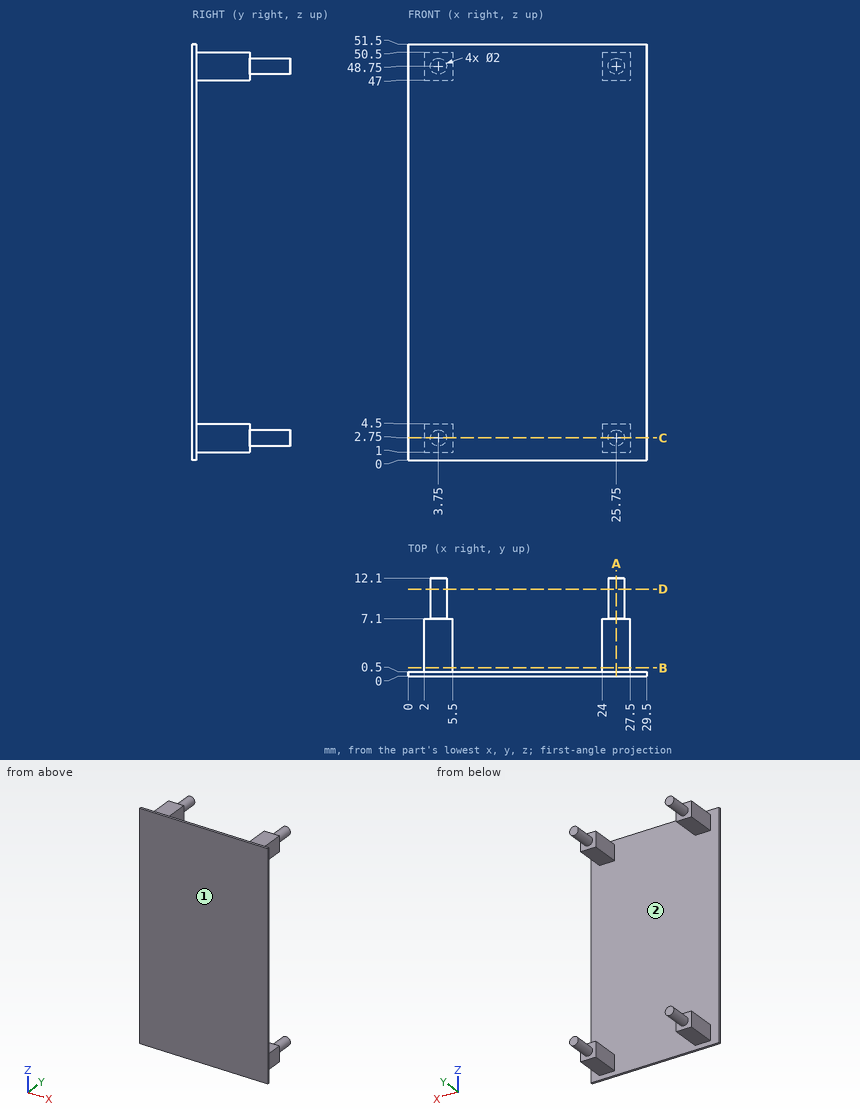
For this review, use the dimensioned drawing (mm, ordinates from the lowest corner) and the shaded views. Coordinates: 2 decimals unless noted, no trailing zeros. Write each loop counter-clockwise with the first axis right and the second up, starting at its lowest first coordinate (ties: lowest second). Pieces come first, ordered by that corner, then holes. Notation, with made-up numbers: (89, 0.25) - (98, 0.25) arc R28 ccw to (98, 25.25) - close; hole circle Ø8 at (-18, 26.5). An arc over 180 degrees is marked (long way). Answer in a Markdown table with one row per item. Add a question column.
Q1. Consider section C-C on z = 2.75. Give the boundary of the cut face in (x, y).
Q2. Clearance check with flat-ended pins moving along their axes: pin 1 (9 mm diameter, centred on x = 11.5, z = 38, fed in from +Y); pin 2 (1 mm diameter, centred on x = 25, y = 4.5, fed in from +Z); pin 3 (2 mm diameter, centred on x = 17, y = 3, fed in from +Z); pin 4 (4 mm diameter, centred on y = 4, z = 2, fed in from +X). State where each tip first meets the part, or that it passes through.
Q3. To check wall thickness, follow line 1 along Y through (x, z) = (24, 14.5); line 2 along Z through (x, y) = (3.5, 8); line 3 along X through (y, z) = (8.5, 49.5). State the ranges of each line that lie inside material, in increasing order. Write a range as from..to.
Q4. Consider section D-D on y = 10.75. Give the boundary of the cut face in (x, z), then the cut area to 3 significant figures.
Q5. Draft analysis for pull direction Z (two halves, no side actions). For the marked faces 1 and 2, state which applies: +Z half, -Z half, draft (parallel to the pull), parting line (faces both ways), or undercut.
Q6. Consider section A-A on x = 25.75. Give the boundary of the cut face in (y, z).
Q7. Consider section B-B on y = 1. Give the boundary of the cut face in (x, z).
Answers below:
| question | item | result |
|---|---|---|
| 1 | outline | (0, 0) - (29.5, 0) - (29.5, 0.5) - (27.5, 0.5) - (27.5, 7.1) - (26.75, 7.1) - (26.75, 12.1) - (24.75, 12.1) - (24.75, 7.1) - (24, 7.1) - (24, 0.5) - (5.5, 0.5) - (5.5, 7.1) - (4.75, 7.1) - (4.75, 12.1) - (2.75, 12.1) - (2.75, 7.1) - (2, 7.1) - (2, 0.5) - (0, 0.5) - close |
| 2 | pin 1 | y = 0.5 |
| 2 | pin 2 | z = 50.5 |
| 2 | pin 3 | through |
| 2 | pin 4 | x = 27.5 |
| 3 | line 1 | 0..0.5 |
| 3 | line 2 | 1.78..3.72, 47.78..49.72 |
| 3 | line 3 | 3.09..4.41, 25.09..26.41 |
| 4 | outline | circle Ø2 at (3.75, 2.75); circle Ø2 at (3.75, 48.75); circle Ø2 at (25.75, 2.75); circle Ø2 at (25.75, 48.75) |
| 4 | area | 12.6 mm² |
| 5 | face 1 | draft |
| 5 | face 2 | undercut |
| 6 | outline | (0, 0) - (0.5, 0) - (0.5, 1) - (7.1, 1) - (7.1, 1.75) - (12.1, 1.75) - (12.1, 3.75) - (7.1, 3.75) - (7.1, 4.5) - (0.5, 4.5) - (0.5, 47) - (7.1, 47) - (7.1, 47.75) - (12.1, 47.75) - (12.1, 49.75) - (7.1, 49.75) - (7.1, 50.5) - (0.5, 50.5) - (0.5, 51.5) - (0, 51.5) - close |
| 7 | outline | (2, 1) - (5.5, 1) - (5.5, 4.5) - (2, 4.5) - close; (2, 47) - (5.5, 47) - (5.5, 50.5) - (2, 50.5) - close; (24, 1) - (27.5, 1) - (27.5, 4.5) - (24, 4.5) - close; (24, 47) - (27.5, 47) - (27.5, 50.5) - (24, 50.5) - close |
